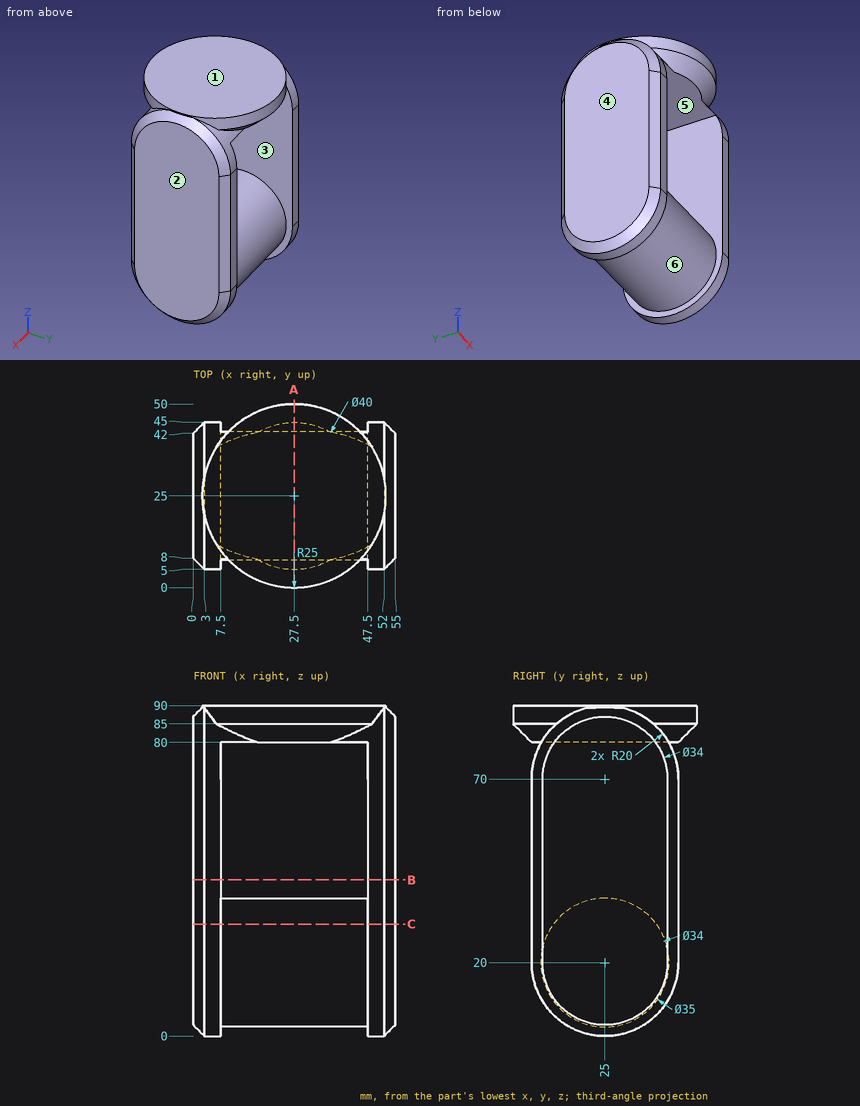
Part print with two shaded views. Sizes in mm from the minimum x, y, z corner. A direction names the side the tool comes from. Round coordinates to 2 decimals unless told otherwise and drop trailing zeros. Order: outer loops, then holes, each group sorted by start corner. A loop starts at its lowest first (then second) coordinate and runs counter-clockwise, first axis right, second up. Notation, with made-up numbers: (33, 57.5) -> (73, 57.5) arc R16 cw to (73, 87.5) -> close; hole circle Ø3 at (27.5, -3.5). An arc over 180 degrees is marked (long way). One line per question, with ' | ' between items.
Q1. Two-plate mould, pull along X, no slides. Class the marked faces 1, 2 and 3: released by +X, released by -X, zero draft, split by the parting line, or undercut.
Completed:
face 1: zero draft | face 2: released by +X | face 3: undercut
Q2. Probe probe 1 along X at (y, z) = (10, 48.5); probe 2 along Y at (x, z) = (5, 66.5); probe 3 along Z at (x, y) = (47, 17). List the from-to ranges inside material, lowest first.
Completed:
probe 1: x = 0 to 7.5, 47.5 to 55 | probe 2: y = 5 to 45 | probe 3: z = 4.44 to 35.56, 80 to 90
Q3. Which spindle directions (+Z, -Z, +X, -X, +Y, -Y) get a long thin tool onto all of the face, cutting with end or side? Do the marked faces 4, 5 and 6. Say none if no direction does.
Completed:
face 4: +Z, -Z, -X, +Y, -Y | face 5: +Y, -Y | face 6: none
Q4. Drop flat-ended pins along their axis: pin 1 (1.4 mm diameter, centred on x = 4, z = 40, fed in from -Y); pin 2 (12 mm diameter, centred on x = 46, z = 69.5, fed in from +Y); pin 3 (12 mm diameter, centred on x = 16, y = 33, fed in from -Z). Give the stop position or say it passes through.
Completed:
pin 1: stops at y = 5 | pin 2: stops at y = 45 | pin 3: stops at z = 2.61
Q5. Slice it at C-C (z = 30.5). Write the cut outline in (x, y), then the cut area to 3 significant figures.
Completed:
outline: (0, 8) -> (3, 5) -> (7.5, 5) -> (7.5, 11) -> (47.5, 11) -> (47.5, 5) -> (52, 5) -> (55, 8) -> (55, 42) -> (52, 45) -> (47.5, 45) -> (47.5, 39) -> (7.5, 39) -> (7.5, 45) -> (3, 45) -> (0, 42) -> close | area: 1,700 mm^2
Q6. Slice it at B-B (z = 42.5). Write the cut outline in (x, y).
Completed:
outline: (0, 8) -> (3, 5) -> (7.5, 5) -> (7.5, 45) -> (3, 45) -> (0, 42) -> close; (47.5, 5) -> (52, 5) -> (55, 8) -> (55, 42) -> (52, 45) -> (47.5, 45) -> close
Q7. Slice it at A-A (x = 27.5). Write the cut outline in (y, z).
Completed:
outline: (0, 85) -> (5, 80) -> (45, 80) -> (50, 85) -> (50, 90) -> (0, 90) -> close; circle Ø35 at (25, 20)
